Read the model definition and answer for the solid it produces. Units are mm, in the model's axes. A direction names the side the tool comes from. Round coordinates to 2 decimals unless told otherwise and drop trailing zeros. Write each loop counter-clockwise with the first axis right and the second up, starting at its lowest first coordinate (ties: lowest second). Pieces come first, ordered by that corner, then holes. Notation, with made-up numbers: (53.25, 46.5) - (62.25, 46.5) arc R24 cw to (62.25, 71.5) - close; hole circle Ø6 at (84.5, -9). An arc over 180 degrees is marked (long way). Answer as CSV lines item,"result". Start each with the question number.
1) Which of the six approach directions +Z, -Z, +X, -X, +Y, -Y give full straight-line access (tool end or side, diameter ignored) to faces 1 (the cylindrical face through (3.451, 41.785, -0.234)), 2 (the flat face through (7, -10, -30))?
2) Find section A-A on y = 0. Determine the outline of the cut face in (x, z).
3) Each of these flat-tipped pins is pushed along its axis until it touches: pin 1 (6 mm diameter, centred on x = 9, y = -11, fed in from -Z); pin 2 (6 mm diameter, centred on x = 8, y = -24.5, fed in from -Z); pin 3 (6 mm diameter, centred on x = 3.5, z = 34.5, fed in from +Y). Where does it stop, or does it pass through?
4) Find section B-B on x = 2.75. Determine the outline of the cut face in (y, z).
5) Find section C-C on z = 40. Determine the outline of the cut face in (x, y).
6) For a pull along Z with two mould halves and no side action, classify faces 3 (the flat face through (10, -14, -25)), 4 (the cylindrical face through (3.45, 45.61, 5.99)), 5 (the flat face through (5, 13, -12)) as +Z half, -Z half, draft (parallel to the pull), parting line (faces both ways), or undercut.
7) Consider line 1 along Y through (x, z) = (2.25, 0); line 2 along Y through (x, z) = (5.25, 0); line 3 along Z through (x, y) = (4.5, -8). Determine where each line is inside the solid, lowest interval first.
from build123d import *

# Parameters (mm, degrees)
SKETCH_1_R          = 46
SKETCH_1_R_2        = 17.5
EXTRUDE_1_DEPTH     = 5
SKETCH_2_R          = 31
SKETCH_2_R_2        = 28.5
EXTRUDE_2_DEPTH     = 5
SKETCH_4_R          = 46
SKETCH_4_R_2        = 31
EXTRUDE_3_DEPTH     = 2
SKETCH_5_R          = 1.8
CUT_EXTRUDE_1_DEPTH = 7


with BuildPart() as part:
    # 草图1 → 凸台-拉伸1 (new body)
    with BuildSketch(Plane(origin=(0, 0, 0), x_dir=(0, 0, -1), z_dir=(1, 0, 0))):
        Circle(SKETCH_1_R)
        Circle(SKETCH_1_R_2, mode=Mode.SUBTRACT)
    extrude(amount=EXTRUDE_1_DEPTH)

    # 草图2 → 凸台-拉伸2 (add)
    with BuildSketch(Plane(origin=(5, 0, 0), x_dir=(0, 0, -1), z_dir=(1, 0, 0))):
        Circle(SKETCH_2_R)
        Circle(SKETCH_2_R_2, mode=Mode.SUBTRACT)
    extrude(amount=EXTRUDE_2_DEPTH)

    # 草图4 → 凸台-拉伸3 (add)
    with BuildSketch(Plane(origin=(5, 0, 0), x_dir=(0, 0, -1), z_dir=(1, 0, 0))):
        Circle(SKETCH_4_R)
        Circle(SKETCH_4_R_2, mode=Mode.SUBTRACT)
    extrude(amount=EXTRUDE_3_DEPTH)

    # 草图5 → 切除-拉伸1 (cut)
    with BuildSketch(Plane.ZY):
        with Locations((0, 40)):
            Circle(SKETCH_5_R)
        with Locations((40, 0)):
            Circle(SKETCH_5_R)
        with Locations((0, -40)):
            Circle(SKETCH_5_R)
        with Locations((-40, 0)):
            Circle(SKETCH_5_R)
    extrude(amount=-CUT_EXTRUDE_1_DEPTH, mode=Mode.SUBTRACT)


solid = part.part
Check values:
1,face 1,"+X, -X"
1,face 2,"+X"
2,outline,"(0, -46) - (7, -46) - (7, -41.8) - (0, -41.8) - close; (0, -38.2) - (7, -38.2) - (7, -31) - (10, -31) - (10, -28.5) - (5, -28.5) - (5, -17.5) - (0, -17.5) - close; (0, 17.5) - (5, 17.5) - (5, 28.5) - (10, 28.5) - (10, 31) - (7, 31) - (7, 38.2) - (0, 38.2) - close; (0, 41.8) - (7, 41.8) - (7, 46) - (0, 46) - close"
3,pin 1,"stops at z = -45.16"
3,pin 2,"stops at z = -40.58"
3,pin 3,"stops at y = 33.52"
4,outline,"circle Ø92 at (0, 0); hole circle Ø3.6 at (-40, 0); hole circle Ø35 at (0, 0); hole circle Ø3.6 at (0, -40); hole circle Ø3.6 at (0, 40); hole circle Ø3.6 at (40, 0)"
5,outline,"(0, -22.72) - (7, -22.72) - (7, -1.8) - (0, -1.8) - close; (0, 1.8) - (7, 1.8) - (7, 22.72) - (0, 22.72) - close"
6,face 3,"draft"
6,face 4,"parting line"
6,face 5,"undercut"
7,line 1,"y = -46 to -41.8, -38.2 to -17.5, 17.5 to 38.2, 41.8 to 46"
7,line 2,"y = -46 to -41.8, -38.2 to -28.5, 28.5 to 38.2, 41.8 to 46"
7,line 3,"z = -45.3 to -15.56, 15.56 to 45.3"
